Drawing for the job (mm, zero at the part's lowest x, y, z). Give positions to 0.01 mm unless a question says otherwise; leave off trailing zeros. Order: outer loops, then holes, each group sorted by start corner. A loop starts at its lowest first (then second) coordinate and runs counter-clockwise, first axis right, second up. Notation, with made-up numbers: (19.25, 54) - (47.25, 54) arc R36 ccw to (47.25, 88) - close; hole circle Ø6 at (81.25, 4). An arc over 180 degrees is marked (long way). One line per item, written item: value.
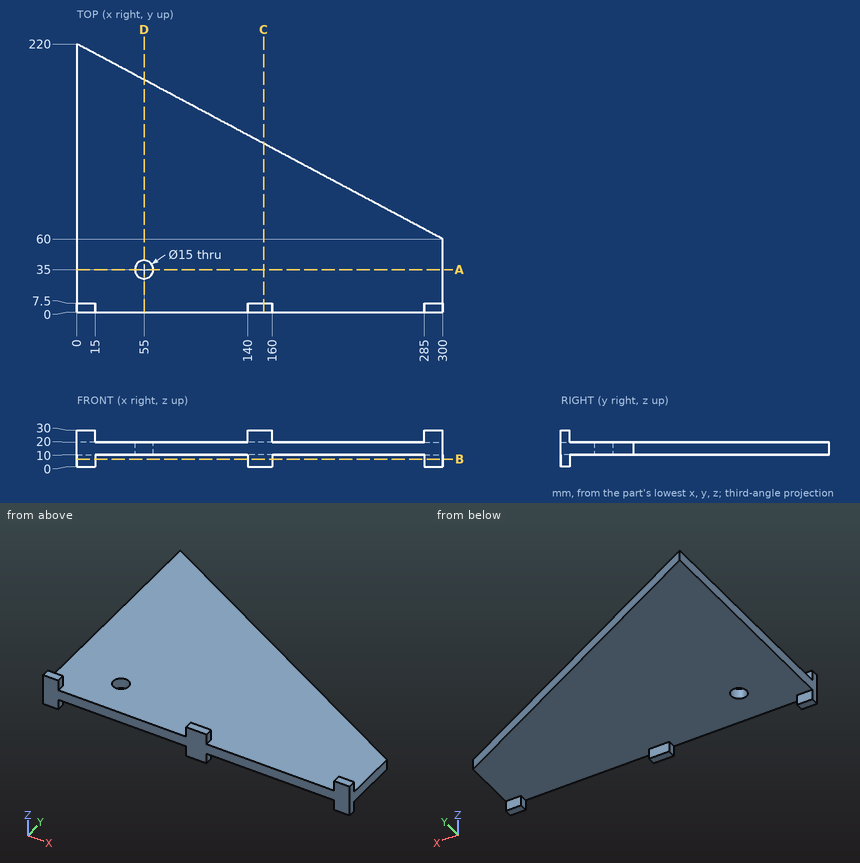
(1) Slice it at B-B, the plane z = 6.25. Give the cut face in (x, y), and give its area (3 significant figures).
Completed:
outline: (0, 0) - (15, 0) - (15, 7.5) - (0, 7.5) - close; (140, 0) - (160, 0) - (160, 7.5) - (140, 7.5) - close; (285, 0) - (300, 0) - (300, 7.5) - (285, 7.5) - close
area: 375 mm²
(2) Slice it at A-A, the plane y = 35. Give the cut face in (x, z), and give its area (3 significant figures).
Completed:
outline: (0, 10) - (47.5, 10) - (47.5, 20) - (0, 20) - close; (62.5, 10) - (300, 10) - (300, 20) - (62.5, 20) - close
area: 2,850 mm²
(3) Slice it at D-D, the plane x = 55. Give the cut face in (y, z).
Completed:
outline: (0, 10) - (27.5, 10) - (27.5, 20) - (0, 20) - close; (42.5, 10) - (190.67, 10) - (190.67, 20) - (42.5, 20) - close
(4) Pin check, flat tips, straight feed: P1, Ø3, axis at y = 191, z = 16, coming from the +X side; P2, Ø1, axis at x = 72, y = 173, coming from the +Z side; P3, Ø1, axis at x = 178.5, y = 119, coming from the -Z side. Stop position of each tip, or through.
Completed:
P1: x = 57.19
P2: z = 20
P3: z = 10
(5) Drill centre lines: line 1 (Z direction, x = 108.5, y = 94); line 2 (X direction, y = 36.5, z = 14.75); line 3 (Y direction, x = 55, z = 17.5). Where is each one in solid material? Low to high.
Completed:
line 1: 10 to 20
line 2: 0 to 47.65, 62.35 to 300
line 3: 0 to 27.5, 42.5 to 190.67
(6) Slice it at C-C, the plane x = 153. Give the cut face in (y, z), and give its area (3 significant figures).
Completed:
outline: (0, 0) - (7.5, 0) - (7.5, 10) - (138.4, 10) - (138.4, 20) - (7.5, 20) - (7.5, 30) - (0, 30) - close
area: 1,530 mm²
